Model file for the job. Use its own axes, mm. Face numbers are marked on the shaded views. A direction names the side the tool comes from. Give positions to 0.01 mm unless a question says otherwise; leave off trailing zeros. Loops run counter-clockwise (first coordinate to the right, second up) from the corner with the lowest first, then second, coordinate; pieces in that order, holes last. Notation, with made-up numbers: (23, 6) - (81, 6) arc R12 ccw to (81, 14) - close; hole circle Ø7 at (87.25, 60). An arc over 180 degrees is marked (long way). Answer as CSV lines item,"result". Start each with the question number.
Item 1: Saw through at C-C on y = 5.5. State how many separate pieces and enclosed holes the cut face has, plus the area to 3 significant figures.
Item 2: Tool access for the marked faces 1 and 2: list every direction of +Z, -Z, +X, -X, +Y, -Y with a clear straight run to the whole face (end or side of a thin tool).
Item 3: Saw through at D-D on z = 31.5. Give the cut face in (x, y), plus the area to 3 significant figures.
Item 4: Saw through at A-A on z = -62. Give the cut face in (x, y), plus the area to 3 significant figures.
Item 5: Pin check, flat tips, straight feed: pin 1 (4.5 mm diameter, centred on y = 7.5, z = -63.5, fed in from +X); pin 2 (1.8 mm diameter, centred on x = -42, y = 9, fed in from -Z); pin 3 (13.5 mm diameter, centred on y = 14.5, z = 79.5, fed in from +X). Stop position of each tip, or through.
Item 6: Saw through at B-B on x = 38. Give the cut face in (y, z), plus the area to 3 significant figures.
Item 7: Pull direction Z, two halves, no side cores. Call the marked faces 3, 4 and 5: pulls with the +Z half, pulls with the -Z half, needs draft (parallel to the pull), parting line crosses it, or undercut.
Item 8: Drill centre lines: L1, parallel to X at y = 9, z = 81; L2, parallel to X at y = 23, z = 72; L3, parallel to X at y = 18.5, z = 80. Where is each one in solid material? Low to high. Write a range as from..to.
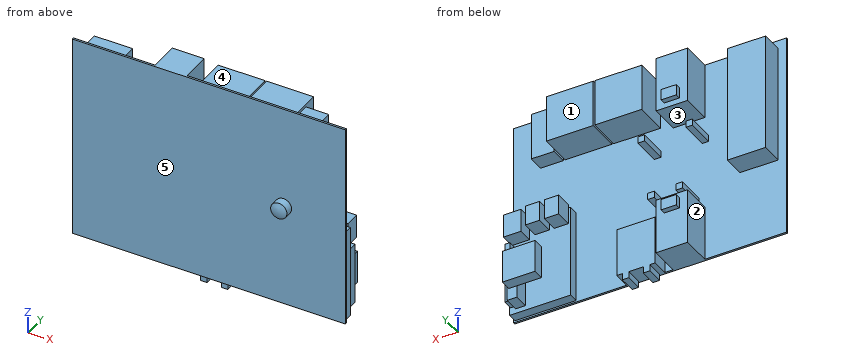
Autodesk Inventor part; units mm, degrees
ref_plane "YZ Plane" through (0, 0, 0) normal (1, 0, 0) x (0, 1, 0)
ref_plane "XZ Plane" through (0, 0, 0) normal (0, 1, 0) x (-1, 0, 0)
ref_plane "XY Plane" through (0, 0, 0) normal (0, 0, 1) x (1, 0, 0)
sketch "Esquisse1" plane through (0, 0, 0) normal (0, 1, 0) x (-1, 0, 0)
  line L0 (125.5, 94.5) -> (-125.5, 94.5)
  line L1 (-125.5, 94.5) -> (-125.5, -94.5)
  line L2 (-125.5, -94.5) -> (125.5, -94.5)
  line L3 (125.5, -94.5) -> (125.5, 94.5)
  line L4 (125.5, 94.5) -> (-125.5, -94.5) construction
  line L5 (-125.5, 94.5) -> (125.5, -94.5) construction
  point P0 (0, 0)
  dimension "d0" = 251
  dimension "d1" = 189
extrude "Extrusion1" add sketch "Esquisse1" along normal blind 1.8
sketch "Esquisse2" plane through (0, 1.8, 0) normal (0, 1, 0) x (1, 0, 0)
  line L0 (124, 93) -> (67.9, 93)
  line L1 (67.9, 93) -> (67.9, 7.5)
  line L2 (67.9, 7.5) -> (124, 7.5)
  line L3 (124, 7.5) -> (124, 93)
  line L4 (125.5, 94.5) -> (-125.5, 94.5)
  line L5 (125.5, -94.5) -> (125.5, 94.5)
  point P0 (0, 0)
  dimension "d4" = 1.5
  dimension "d5" = 1.5
  dimension "d6" = 56.1
  dimension "d7" = 85.5
extrude "Extrusion2" add sketch "Esquisse2" along normal blind 8.7
sketch "Esquisse3" plane through (0, 10.5, 0) normal (0, 1, 0) x (1, 0, 0)
  line L0 (121.8, 25.8) -> (105.8, 25.8)
  line L1 (105.8, 25.8) -> (105.8, 4.4)
  line L2 (105.8, 4.4) -> (121.8, 4.4)
  line L3 (121.8, 4.4) -> (121.8, 25.8)
  line L4 (124, 7.5) -> (124, 93)
  line L5 (67.9, 7.5) -> (124, 7.5)
  point P0 (0, 0)
  dimension "d10" = 21.4
  dimension "d11" = 16
  dimension "d12" = 2.2
  dimension "d13" = 3.1
extrude "Extrusion3" add sketch "Esquisse3" along normal blind 13.5
sketch "Esquisse4" plane through (0, 10.5, 0) normal (0, 1, 0) x (1, 0, 0)
  line L0 (69.9, 22.7) -> (83, 22.7)
  line L1 (83, 22.7) -> (83, 4.4)
  line L2 (83, 4.4) -> (69.9, 4.4)
  line L3 (69.9, 4.4) -> (69.9, 22.7)
  line L4 (67.9, 93) -> (67.9, 7.5)
  line L5 (105.8, 4.4) -> (121.8, 4.4)
  line L6 (87.5, 4.4) -> (100.6, 4.4)
  line L7 (100.6, 4.4) -> (100.6, 22.7)
  line L8 (100.6, 22.7) -> (87.5, 22.7)
  line L9 (87.5, 22.7) -> (87.5, 4.4)
  point P0 (0, 0)
  point P1 (76.45, 4.4)
  point P2 (76.45, 22.7)
  dimension "d16" = 13.1
  dimension "d17" = 18.3
  dimension "d18" = 2
  dimension "d19" = 4.5
  dimension "d20" = 13.1
extrude "Extrusion4" add sketch "Esquisse4" along normal blind 15.5
sketch "Esquisse5" plane through (0, 10.5, 0) normal (0, 1, 0) x (1, 0, 0)
  line L0 (123, 86) -> (118.5, 86)
  line L1 (118.5, 86) -> (118.5, 29.6)
  line L2 (118.5, 29.6) -> (123, 29.6)
  line L3 (123, 29.6) -> (123, 86)
  line L4 (124, 7.5) -> (124, 93)
  line L5 (124, 93) -> (67.9, 93)
  point P0 (0, 0)
  dimension "d23" = 56.4
  dimension "d24" = 4.5
  dimension "d25" = 1
  dimension "d26" = 7
extrude "Extrusion5" add sketch "Esquisse5" along normal blind 9
sketch "Esquisse6" plane through (0, 10.5, 0) normal (0, 1, 0) x (1, 0, 0)
  line L0 (118.5, 29.6) -> (118.5, 86)
  line L1 (118.5, 86) -> (118.5, 88.7)
  line L2 (118.5, 88.7) -> (109.5, 88.7)
  line L3 (109.5, 88.7) -> (109.5, 47.7)
  line L4 (109.5, 47.7) -> (118.5, 47.7)
  line L5 (124, 93) -> (67.9, 93)
  point P0 (0, 0)
  dimension "d29" = 9
  dimension "d30" = 41
  dimension "d31" = 4.3
extrude "Extrusion6" add sketch "Esquisse6" along normal blind 13.6
sketch "Esquisse7" plane through (0, 24.1, 0) normal (0, 1, 0) x (1, 0, 0)
  line L0 (118.5, 47.7) -> (109.5, 47.7)
  line L1 (116.8, 47.7) -> (86.8, 47.7)
  line L2 (86.8, 47.7) -> (86.8, 77.7)
  line L3 (86.8, 77.7) -> (116.8, 77.7)
  line L4 (116.8, 77.7) -> (116.8, 47.7)
  line L5 (118.5, 47.7) -> (118.5, 88.7)
  point P0 (0, 0)
  dimension "d34" = 30
  dimension "d35" = 30
  dimension "d36" = 1.7
extrude "Extrusion7" add sketch "Esquisse7" along normal blind 10.3
sketch "Esquisse8" plane through (0, 1.8, 0) normal (0, 1, 0) x (1, 0, 0)
  line L0 (125.5, 94.5) -> (-125.5, 94.5)
  line L1 (-50.4, 94.5) -> (-21.3, 94.5)
  line L2 (-21.3, 94.5) -> (-21.3, 43.5)
  line L3 (-21.3, 43.5) -> (-50.4, 43.5)
  line L4 (-50.4, 43.5) -> (-50.4, 94.5)
  line L5 (-125.5, 94.5) -> (-125.5, -94.5)
  point P0 (0, 0)
  dimension "d39" = 75.1
  dimension "d40" = 29.1
  dimension "d41" = 51
extrude "Extrusion8" add sketch "Esquisse8" along normal blind 27.3
sketch "Esquisse9" plane through (0, 29.1, 0) normal (0, 1, 0) x (1, 0, 0)
  line L0 (-28.85, 48.5) -> (-42.85, 48.5)
  line L1 (-42.85, 48.5) -> (-42.85, 58.5)
  line L2 (-42.85, 58.5) -> (-28.85, 58.5)
  line L3 (-28.85, 58.5) -> (-28.85, 48.5)
  line L4 (-21.3, 43.5) -> (-21.3, 94.5)
  line L5 (-50.4, 94.5) -> (-50.4, 43.5)
  line L6 (-21.3, 94.5) -> (-50.4, 94.5)
  point P0 (0, 0)
  dimension "d44" = 10
  dimension "d45" = 14
  dimension "d46" = 7.55
  dimension "d47" = 7.55
  dimension "d48" = 36
extrude "Extrusion9" add sketch "Esquisse9" along normal blind 5
mirror "Symétrie1" about plane through (0, 0, 0) normal (0, 0, 1) of "Extrusion8", "Extrusion9"
sketch "Esquisse10" plane through (0, 1.8, 0) normal (0, 1, 0) x (1, 0, 0)
  line L0 (125.5, 94.5) -> (-21.3, 94.5)
  line L1 (-13.8, 94.5) -> (21.4, 94.5)
  line L2 (21.4, 94.5) -> (21.4, 50)
  line L3 (21.4, 50) -> (-13.8, 50)
  line L4 (-13.8, 50) -> (-13.8, 94.5)
  line L5 (16.4, 94.5) -> (10.4, 94.5)
  line L6 (10.4, 94.5) -> (10.4, 100.5)
  line L7 (10.4, 100.5) -> (16.4, 100.5)
  line L8 (16.4, 100.5) -> (16.4, 94.5)
  line L9 (-2.8, 94.5) -> (-8.8, 94.5)
  line L10 (-8.8, 94.5) -> (-8.8, 100.5)
  line L11 (-8.8, 100.5) -> (-2.8, 100.5)
  line L12 (-2.8, 100.5) -> (-2.8, 94.5)
  line L13 (-21.3, 43.5) -> (-21.3, 94.5)
  point P0 (0, 0)
  point P1 (21.4, 94.5)
  point P2 (-2.8, 94.5)
  point P3 (-8.8, 94.5)
  dimension "d51" = 44.5
  dimension "d52" = 35.2
  dimension "d53" = 6
  dimension "d54" = 6
  dimension "d55" = 6
  dimension "d56" = 5
  dimension "d57" = 5
  dimension "d115" = 7.5
extrude "Extrusion10" add sketch "Esquisse10" along normal blind 15.5
sketch "Esquisse11" plane through (0, 1.8, 0) normal (0, 1, 0) x (1, 0, 0)
  line L0 (-9.8, -90.5) -> (33.3, -90.5)
  line L1 (33.3, -90.5) -> (33.3, -47.4)
  line L2 (33.3, -47.4) -> (-9.8, -47.4)
  line L3 (-9.8, -47.4) -> (-9.8, -90.5)
  line L4 (34.8, -90.5) -> (77.9, -90.5)
  line L5 (77.9, -90.5) -> (77.9, -47.4)
  line L6 (77.9, -47.4) -> (34.8, -47.4)
  line L7 (34.8, -47.4) -> (34.8, -90.5)
  line L8 (-21.3, -94.5) -> (125.5, -94.5)
  line L9 (-21.3, -43.5) -> (-21.3, -94.5)
  point P0 (0, 0)
  dimension "d60" = 43.1
  dimension "d61" = 43.1
  dimension "d62" = 43.1
  dimension "d63" = 4
  dimension "d64" = 1.5
  dimension "d65" = 11.5
extrude "Extrusion11" add sketch "Esquisse11" along normal blind 30
sketch "Esquisse12" plane through (0, 1.8, 0) normal (0, 1, 0) x (1, 0, 0)
  line L0 (-117.8, -86.9) -> (-82.8, -86.9)
  line L1 (-82.8, -86.9) -> (-82.8, 21.6)
  line L2 (-82.8, 21.6) -> (-117.8, 21.6)
  line L3 (-117.8, 21.6) -> (-117.8, -86.9)
  line L4 (-125.5, -94.5) -> (-50.4, -94.5)
  line L5 (-125.5, 94.5) -> (-125.5, -94.5)
  point P0 (0, 0)
  dimension "d68" = 108.5
  dimension "d69" = 35
  dimension "d70" = 7.6
  dimension "d71" = 7.7
extrude "Extrusion12" add sketch "Esquisse12" along normal blind 20
sketch "Esquisse13" plane through (0, 1.8, 0) normal (0, 1, 0) x (1, 0, 0)
  line L0 (-21.3, -43.5) -> (-21.3, -94.5)
  line L1 (-4, -25) -> (-10, -25)
  line L2 (-10, -25) -> (-10, -19)
  line L3 (-10, -19) -> (-4, -19)
  line L4 (-4, -19) -> (-4, -25)
  line L5 (-4, -25) -> (-10, -19) construction
  line L6 (-10, -25) -> (-4, -19) construction
  line L7 (-48, -25) -> (-54, -25)
  line L8 (-54, -25) -> (-54, -19)
  line L9 (-54, -19) -> (-48, -19)
  line L10 (-48, -19) -> (-48, -25)
  line L11 (-48, -25) -> (-54, -19) construction
  line L12 (-54, -25) -> (-48, -19) construction
  line L13 (-7, -22) -> (-51, -22)
  line L14 (-125.5, -94.5) -> (-50.4, -94.5)
  line L15 (-125.5, 94.5) -> (-125.5, -94.5)
  line L16 (-39, 33) -> (-45, 33)
  line L17 (-45, 33) -> (-45, 39)
  line L18 (-45, 39) -> (-39, 39)
  line L19 (-39, 39) -> (-39, 33)
  line L20 (-39, 33) -> (-45, 39) construction
  line L21 (-45, 33) -> (-39, 39) construction
  line L22 (-42, 36) -> (-16, 36)
  line L23 (-13, 33) -> (-19, 33)
  line L24 (-19, 33) -> (-19, 39)
  line L25 (-19, 39) -> (-13, 39)
  line L26 (-13, 39) -> (-13, 33)
  line L27 (-13, 33) -> (-19, 39) construction
  line L28 (-19, 33) -> (-13, 39) construction
  point P0 (0, 0)
  dimension "d87" = 6
  dimension "d88" = 6
  dimension "d89" = 6
  dimension "d90" = 6
  dimension "d91" = 72.5
  dimension "d92" = 74.5
  dimension "d93" = 44
  dimension "d94" = 6
  dimension "d95" = 6
  dimension "d96" = 6
  dimension "d97" = 6
  dimension "d98" = 58
  dimension "d99" = 9
  dimension "d101" = 26
  dimension "d102" = 9
extrude "Extrusion13" add sketch "Esquisse13" along normal blind 26
sketch "Esquisse14" plane through (0, 0, 0) normal (0, 0, 1) x (1, 0, 0)
  line L0 (125.5, 0) -> (-125.5, 0)
  line L1 (76, 0) -> (76, -7.4346)
  line L2 (68.5, 0) -> (68.5, -9.1)
  arc A0 (68.5, -9.1) -> (76, -7.4346) centre (68.5, 8.6202) ccw
  line L3 (125.5, 0) -> (125.5, 1.8)
  point P0 (0, 0)
  dimension "d105" = 9.1
  dimension "d106" = 7.5
  dimension "d107" = 49.5
revolve "Révolution1" add sketch "Esquisse14" angle 360 about axis through (68.5, 0, 0) along (0, -1, 0)
sketch "Esquisse15" plane through (0, 1.8, 0) normal (0, 1, 0) x (1, 0, 0)
  line L0 (79.6, -90.5) -> (100.5, -90.5)
  line L1 (100.5, -90.5) -> (100.5, -47.3)
  line L2 (100.5, -47.3) -> (79.6, -47.3)
  line L3 (79.6, -47.3) -> (79.6, -90.5)
  line L4 (-21.3, -94.5) -> (125.5, -94.5)
  line L5 (34.8, -90.5) -> (77.9, -90.5)
  line L6 (77.9, -90.5) -> (77.9, -47.4)
  point P0 (0, 0)
  dimension "d109" = 20.9
  dimension "d110" = 43.2
  dimension "d112" = 1.7
extrude "Extrusion14" add sketch "Esquisse15" along normal blind 14.8
equation "\"d5\" = d4"
equation "\"d20\" = d16"
equation "\"d35\" = d34"
equation "\"d46\" = d47"
equation "\"d54\" = d53"
equation "\"d55\" = d53"
equation "\"d57\" = d56"
equation "\"d61\" = d60"
equation "\"d62\" = d60"
equation "\"d88\" = d87"
equation "\"d89\" = d88"
equation "\"d90\" = d87"
equation "\"d94\" = d88"
equation "\"d95\" = d94"
equation "\"d96\" = d95"
equation "\"d97\" = d94"
equation "\"d99\" = d102"
Responses:
1,separate pieces,"12"
1,enclosed holes,"0"
1,area,"18,000 mm2"
2,face 1,"+Z, -Z, +X, +Y"
2,face 2,"-Z, -X, +Y"
3,outline,"(-125.5, 0) - (125.5, 0) - (125.5, 1.8) - (-82.8, 1.8) - (-82.8, 21.8) - (-117.8, 21.8) - (-117.8, 1.8) - (-125.5, 1.8) - close"
3,area,"1,150 mm2"
4,outline,"(-125.5, 0) - (125.5, 0) - (125.5, 1.8) - (124, 1.8) - (124, 10.5) - (123, 10.5) - (123, 19.5) - (118.5, 19.5) - (118.5, 24.1) - (116.8, 24.1) - (116.8, 34.4) - (86.8, 34.4) - (86.8, 24.1) - (109.5, 24.1) - (109.5, 10.5) - (67.9, 10.5) - (67.9, 1.8) - (21.4, 1.8) - (21.4, 17.3) - (-13.8, 17.3) - (-13.8, 1.8) - (-21.3, 1.8) - (-21.3, 29.1) - (-50.4, 29.1) - (-50.4, 1.8) - (-125.5, 1.8) - close"
4,area,"2,750 mm2"
5,pin 1,"x = 124"
5,pin 2,"z = -94.5"
5,pin 3,"x = 100.5"
6,outline,"(0, -94.5) - (1.8, -94.5) - (1.8, 47.4) - (31.8, 47.4) - (31.8, 90.5) - (1.8, 90.5) - (1.8, 94.5) - (0, 94.5) - close"
6,area,"1,630 mm2"
7,face 3,"undercut"
7,face 4,"pulls with the +Z half"
7,face 5,"needs draft"
8,L1,"-117.8..-82.8, -50.4..-21.3, -9.8..33.3, 34.8..77.9, 79.6..100.5"
8,L2,"-50.4..-21.3, -9.8..33.3, 34.8..77.9"
8,L3,"-117.8..-82.8, -50.4..-21.3, -9.8..33.3, 34.8..77.9"
